from build123d import *

# Parameters (mm, degrees)
SKETCH1_W           = 52
SKETCH1_H           = 23.5
SKETCH1_W_2         = 21.5
SKETCH1_H_2         = 25
BOSS_EXTRUDE1_DEPTH = 2
CUT_EXTRUDE1_DEPTH  = 2
SKETCH3_R           = 2
CUT_EXTRUDE2_DEPTH  = 10


with BuildPart() as part:
    # Sketch1 → Boss-Extrude1 (new body)
    with BuildSketch(Plane.XY):
        with Locations((0, 24.25)):
            Rectangle(SKETCH1_W, SKETCH1_H)
        with BuildLine():
            Line((26, 36), (26, 12.5))
            Line((26, 12.5), (47.5, 12.5))
            ThreePointArc((47.5, 12.5), (41.925608309, 28.985131006), (26, 36))
        make_face()
        with Locations((36.75, 0)):
            Rectangle(SKETCH1_W_2, SKETCH1_H_2)
        Rectangle(SKETCH1_W, SKETCH1_H_2)
        with BuildLine():
            Line((47.5, -12.5), (26, -12.5))
            Line((26, -12.5), (26, -36))
            ThreePointArc((26, -36), (41.314036989, -28.425608309), (47.5, -12.5))
        make_face()
        with Locations((0, -24.25)):
            Rectangle(SKETCH1_W, SKETCH1_H)
        with BuildLine():
            Line((-26, -12.5), (-47.5, -12.5))
            ThreePointArc((-47.5, -12.5), (-41.925608309, -28.985131006), (-26, -36))
            Line((-26, -36), (-26, -12.5))
        make_face()
        with Locations((-36.75, 0)):
            Rectangle(SKETCH1_W_2, SKETCH1_H_2)
        with BuildLine():
            ThreePointArc((-26, 36), (-41.314036989, 28.425608309), (-47.5, 12.5))
            Line((-47.5, 12.5), (-26, 12.5))
            Line((-26, 12.5), (-26, 36))
        make_face()
    extrude(amount=BOSS_EXTRUDE1_DEPTH)

    # Sketch2 → Cut-Extrude1 (cut)
    with BuildSketch(Plane.XY.offset(2)):
        with BuildLine():
            Line((0, -1.499605822), (-41.5, -1.499605822))
            ThreePointArc((-41.5, -1.499605822), (-43.000394178, -3), (-41.5, -4.500394178))
            Line((-41.5, -4.500394178), (41.5, -4.500394178))
            ThreePointArc((41.5, -4.500394178), (43.000394178, -3), (41.5, -1.499605822))
            Line((41.5, -1.499605822), (0, -1.499605822))
        make_face()
        with BuildLine():
            ThreePointArc((-18, 28.495571567), (-19.495571567, 27), (-18, 25.504428433))
            Line((-18, 25.504428433), (18, 25.504428433))
            ThreePointArc((18, 25.504428433), (19.495571567, 27), (18, 28.495571567))
            Line((18, 28.495571567), (-18, 28.495571567))
        make_face()
        with BuildLine():
            Line((41.5, -7.509541658), (-41.5, -7.509541658))
            ThreePointArc((-41.5, -7.509541658), (-42.990458342, -9), (-41.5, -10.490458342))
            Line((-41.5, -10.490458342), (41.5, -10.490458342))
            ThreePointArc((41.5, -10.490458342), (42.990458342, -9), (41.5, -7.509541658))
        make_face()
        with BuildLine():
            Line((38, -13.507793121), (-38, -13.507793121))
            ThreePointArc((-38, -13.507793121), (-39.492206879, -15), (-38, -16.492206879))
            Line((-38, -16.492206879), (38, -16.492206879))
            ThreePointArc((38, -16.492206879), (39.492206879, -15), (38, -13.507793121))
        make_face()
        with BuildLine():
            Line((28, -19.493656832), (-28, -19.493656832))
            ThreePointArc((-28, -19.493656832), (-29.506343168, -21), (-28, -22.506343168))
            Line((-28, -22.506343168), (0, -22.506343168))
            Line((0, -22.506343168), (28, -22.506343168))
            ThreePointArc((28, -22.506343168), (29.506343168, -21), (28, -19.493656832))
        make_face()
        with BuildLine():
            Line((18, -25.504428433), (-18, -25.504428433))
            ThreePointArc((-18, -25.504428433), (-19.495571567, -27), (-18, -28.495571567))
            Line((-18, -28.495571567), (18, -28.495571567))
            ThreePointArc((18, -28.495571567), (19.495571567, -27), (18, -25.504428433))
        make_face()
        with BuildLine():
            ThreePointArc((-28, 22.506343168), (-29.506343168, 21), (-28, 19.493656832))
            Line((-28, 19.493656832), (28, 19.493656832))
            ThreePointArc((28, 19.493656832), (29.506343168, 21), (28, 22.506343168))
            Line((28, 22.506343168), (0, 22.506343168))
            Line((0, 22.506343168), (-28, 22.506343168))
        make_face()
        with BuildLine():
            ThreePointArc((-38, 16.492206879), (-39.492206879, 15), (-38, 13.507793121))
            Line((-38, 13.507793121), (38, 13.507793121))
            ThreePointArc((38, 13.507793121), (39.492206879, 15), (38, 16.492206879))
            Line((38, 16.492206879), (-38, 16.492206879))
        make_face()
        with BuildLine():
            ThreePointArc((-41.5, 10.490458342), (-42.990458342, 9), (-41.5, 7.509541658))
            Line((-41.5, 7.509541658), (41.5, 7.509541658))
            ThreePointArc((41.5, 7.509541658), (42.990458342, 9), (41.5, 10.490458342))
            Line((41.5, 10.490458342), (-41.5, 10.490458342))
        make_face()
        with BuildLine():
            ThreePointArc((-41.5, 4.500394178), (-43.000394178, 3), (-41.5, 1.499605822))
            Line((-41.5, 1.499605822), (41.5, 1.499605822))
            ThreePointArc((41.5, 1.499605822), (43.000394178, 3), (41.5, 4.500394178))
            Line((41.5, 4.500394178), (-41.5, 4.500394178))
        make_face()
    extrude(amount=-CUT_EXTRUDE1_DEPTH, mode=Mode.SUBTRACT)

    # Sketch3 → Cut-Extrude2 (cut)
    with BuildSketch(Plane.XY.offset(2)):
        with Locations((0, 33)):
            Circle(SKETCH3_R)
        with Locations((-13, -33)):
            Circle(SKETCH3_R)
        with Locations((13, -33)):
            Circle(SKETCH3_R)
    extrude(amount=-CUT_EXTRUDE2_DEPTH, mode=Mode.SUBTRACT)


solid = part.part
Check sheet for the modelled part. Datum: model origin and axes. Units: mm. A direction names the side the tool comes from. Give positions to 0.01 mm unless a question says otherwise; leave off trailing zeros. Write each loop counter-clockwise with the first axis right and the second up, starting at its lowest first coordinate (ties: lowest second). Pieces come first, ordered by that corner, then holes. Notation, with made-up numbers: (-1, 65) -> (56, 65) arc R13 ccw to (56, 82) -> close; hole circle Ø10 at (21.5, 70). An arc over 180 degrees is marked (long way). One line per item, written item: value. Start each with the question number.
Item 1: Section check C-C on x = 9. State how many separate pieces and enclosed holes the cut face has, then the cut area to 3 significant figures.
Item 2: Draft check along Y on faces 1 (the flat face through (47.5, 0, 1)), 2 (the flat face through (0, 36, 1)), 3 (the flat face through (1, 4.5, 1)). Enter one of: +Y half, -Y half, draft (parallel to the pull), parting line (faces both ways), or undercut.
Item 3: Section check A-A on y = -3. Record the cut outline in (x, z).
Item 4: Section check B-B on x = -35. Record the cut outline in (y, z), then the cut area to 3 significant figures.
Item 5: Tool access check on faces 4 (the flat face through (-1, 1, 2)), 5 (the flat face through (-1, -10.49, 1)). Record the directions out of +Z, -Z, +X, -X, +Y, -Y that give a thin tool (end or side, any length) a straight path to the whole face; none if there is none.
Item 6: Section check D-D on y = 9. Record the cut outline in (x, z), then the cut area to 3 significant figures.
Item 7: Gauge pin test, flat ends, axial feed: pin 1 (3 mm diameter, centred on x = 13, y = -33, fed in from +Z); pin 2 (1 mm diameter, centred on y = 2, z = 1, fed in from +X); pin 3 (1 mm diameter, centred on y = 12, z = 0.5, fed in from -X). Record the tip position at first contact, or that the pin passes through.
Item 8: Material ranges on probe 1 along Y at (x, z) = (-40, 0.4); probe 2 along X at (y, z) = (26.5, 1); probe 3 along X at (y, z) = (-2.5, 0.6), recorded low to high. Write a range as from..to.
Results list:
1. separate pieces: 11
1. enclosed holes: 0
1. area: 84.1 mm²
2. face 1: draft
2. face 2: +Y half
2. face 3: undercut
3. outline: (-47.5, 0) -> (-43, 0) -> (-43, 2) -> (-47.5, 2) -> close; (43, 0) -> (47.5, 0) -> (47.5, 2) -> (43, 2) -> close
4. outline: (-34.03, 0) -> (-16.49, 0) -> (-16.49, 2) -> (-34.03, 2) -> close; (-13.51, 0) -> (-10.49, 0) -> (-10.49, 2) -> (-13.51, 2) -> close; (-7.51, 0) -> (-4.5, 0) -> (-4.5, 2) -> (-7.51, 2) -> close; (-1.5, 0) -> (1.5, 0) -> (1.5, 2) -> (-1.5, 2) -> close; (4.5, 0) -> (7.51, 0) -> (7.51, 2) -> (4.5, 2) -> close; (10.49, 0) -> (13.51, 0) -> (13.51, 2) -> (10.49, 2) -> close; (16.49, 0) -> (33.32, 0) -> (33.32, 2) -> (16.49, 2) -> close
4. area: 98.8 mm²
5. face 4: +Z, +X, -X, +Y, -Y
5. face 5: +Z, -Z
6. outline: (-47.5, 0) -> (-42.99, 0) -> (-42.99, 2) -> (-47.5, 2) -> close; (42.99, 0) -> (47.5, 0) -> (47.5, 2) -> (42.99, 2) -> close
6. area: 18.0 mm²
7. pin 1: through
7. pin 2: x = 47.5
7. pin 3: x = -47.5
8. probe 1: -30.84..-10.49, -7.51..-4.5, -1.5..1.5, 4.5..7.51, 10.49..29.75
8. probe 2: -42.9..-19.41, 19.41..43.88
8. probe 3: -47.5..-42.91, 42.91..47.5
